from build123d import *

# Parameters (mm, degrees)
F0_W     = 38.1
F0_H     = 25.4
F1_DEPTH = 12.7
F2_R     = 9.525
F3_DEPTH = 12.701


with BuildPart() as f1:
    # F0 (on Top) → F1 (new body)
    with BuildSketch(Plane.XY):
        Rectangle(F0_W, F0_H)
        with BuildLine():
            Line((19.05, -12.7), (-19.05, -12.7))
            ThreePointArc((-19.05, -12.7), (0, -31.75), (19.05, -12.7))
        make_face()
    extrude(amount=F1_DEPTH)

    # F2 (on face) → F3 (cut, through all)
    with BuildSketch(Plane.XY.offset(12.7)):
        with Locations((0, -12.7)):
            Circle(F2_R)
    extrude(amount=-F3_DEPTH, mode=Mode.SUBTRACT)


solid = f1.part
Verification items for the finished model (mm, model axes). Round coordinates to 2 decimals unless told otherwise and drop trailing zeros. Loops run counter-clockwise (first coordinate to the right, second up) from the corner with the lowest first, then second, coordinate; pieces in that order, holes last. Notation, with made-up numbers: (44, 24) - (57, 24) arc R12 cw to (57, 36) - close; hole circle Ø8 at (84, 78). An arc over 180 degrees is marked (long way). Use a Markdown table: item, result. Add a question column.
1. Thickness scan on probe 1 along Y at (x, z) = (0, 7) (3 decimals); probe 2 along X at (y, z) = (-12.5, 9.25); probe 3 along X at (y, z) = (-4.5, 9). Record the ranges inside material, lowest first. Write a range as [from, to].
2. Gauge pin test, flat ends, axial feed: pin 1 (4 mm diameter, centred on x = 6, z = 4.5, fed in from -Y); pin 2 (1.5 mm diameter, centred on y = -16.5, z = 8, fed in from +X). Record the tip position at first contact, or that the pin passes through.
3. Section check B-B, the plane z = 8.5. Record the boundary of the cut face in (x, y) (3 decimals).
4. Section check D-D, the plane x = -13. Record the boundary of the cut face in (y, z).
5. Section check C-C, the plane y = -18. Record the boundary of the cut face in (x, z).
6. Release check for a two-part mould opening along Y. For faces 1 (the face through (-0.419, -31.745, 6.261)), 2 (the face through (0, 12.7, 6)), 3 (the face through (-1.24, -3.256, 6.439)) record: released by +Y, released by -Y, zero draft, split by the parting line, or undercut.
7. Section check A-A, the plane x = 0. Record the boundary of the cut face in (y, z) (3 decimals).
Checks:
| question | item | result |
|---|---|---|
| 1 | probe 1 | y = [-31.75, -22.225], [-3.175, 12.7] |
| 1 | probe 2 | x = [-19.05, -9.52], [9.52, 19.05] |
| 1 | probe 3 | x = [-19.05, -4.85], [4.85, 19.05] |
| 2 | pin 1 | stops at y = -31.33 |
| 2 | pin 2 | stops at x = 18.8 |
| 3 | outline | (-19.05, -12.7) arc R19.05 ccw to (19.05, -12.7) - (19.05, 12.7) - (-19.05, 12.7) - close; hole circle Ø19.05 at (0, -12.7) |
| 4 | outline | (-26.62, 0) - (12.7, 0) - (12.7, 12.7) - (-26.62, 12.7) - close |
| 5 | outline | (-18.3, 0) - (-7.91, 0) - (-7.91, 12.7) - (-18.3, 12.7) - close; (7.91, 0) - (18.3, 0) - (18.3, 12.7) - (7.91, 12.7) - close |
| 6 | face 1 | released by -Y |
| 6 | face 2 | released by +Y |
| 6 | face 3 | undercut |
| 7 | outline | (-31.75, 0) - (-22.225, 0) - (-22.225, 12.7) - (-31.75, 12.7) - close; (-3.175, 0) - (12.7, 0) - (12.7, 12.7) - (-3.175, 12.7) - close |
